Check sheet for the modelled part. Datum: model origin and axes. Units: mm. Face numbers are marked on the shaded views. A direction names the side the tool comes from. Give positions to 0.01 mm unless a question says otherwise; leave off trailing zeros. Loops run counter-clockwise (first coordinate to the right, second up) from the corner with the lowest first, then second, coordinate; pieces in that order, holes last.
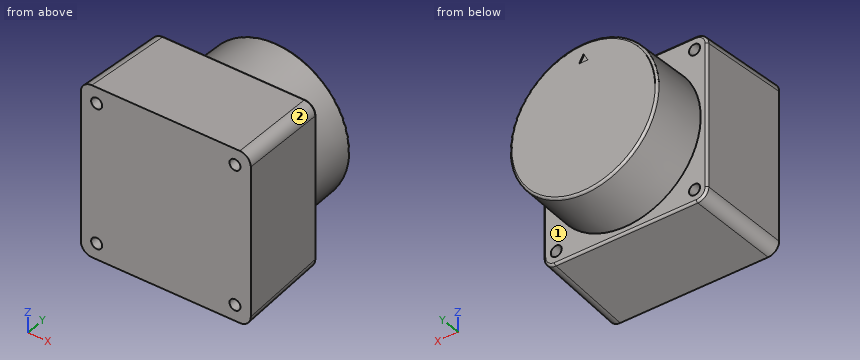
```python
from build123d import *

# Parameters (mm, degrees)
SZKIC1_W                    = 38.59
SZKIC1_H                    = 38.59
SZKIC1_R                    = 1.25
DODANIE_WYCI_GNI_CIE1_DEPTH = 33.3
SZKIC3_OUTSIDE_W            = 53.376
SZKIC3_OUTSIDE_H            = 53.376
SZKIC3_OUTSIDE_R            = 17.645
WYTNIJ_WYCI_GNI_CIE1_DEPTH  = 12.6
POCHYLENIE2_ANGLE           = -2
POCHYLENIE3_ANGLE           = -1.5
ZAOKR_GLENIE2_R             = 2.5
ZAOKR_GLENIE3_R             = 0.5
ZAOKR_GLENIE4_R             = 0.5
WYTNIJ_WYCI_GNI_CIE2_DEPTH  = 0.2


with BuildPart() as part:
    # Szkic1 → Dodanie-wyciągnięcie1 (new body)
    with BuildSketch(Plane(origin=(0, 0, 0), x_dir=(1, 0, 0), z_dir=(0, 1, 0))):
        Rectangle(SZKIC1_W, SZKIC1_H)
        with Locations(Location((-15.7, 15.7, 0), (0, 0, 270))):
            Circle(SZKIC1_R, mode=Mode.SUBTRACT)
        with Locations(Location((15.7, 15.7, 0), (0, 0, 270))):
            Circle(SZKIC1_R, mode=Mode.SUBTRACT)
        with Locations(Location((15.7, -15.7, 0), (0, 0, 270))):
            Circle(SZKIC1_R, mode=Mode.SUBTRACT)
        with Locations(Location((-15.7, -15.7, 0), (0, 0, 270))):
            Circle(SZKIC1_R, mode=Mode.SUBTRACT)
    extrude(amount=DODANIE_WYCI_GNI_CIE1_DEPTH)

    # Szkic3 outside → Wytnij-wyciągnięcie1 (cut)
    with BuildSketch(Plane(origin=(0, 33.3, 0), x_dir=(1, 0, 0), z_dir=(0, 1, 0))):
        Rectangle(SZKIC3_OUTSIDE_W, SZKIC3_OUTSIDE_H)
        with Locations(Location((0, 0, 0), (0, 0, 270))):
            Circle(SZKIC3_OUTSIDE_R, mode=Mode.SUBTRACT)
    extrude(amount=-WYTNIJ_WYCI_GNI_CIE1_DEPTH, mode=Mode.SUBTRACT)

    # Pochylenie2
    pochylenie2_faces = [part.faces().sort_by_distance(p)[0] for p in [
        (19.295, 10.35, 0),
        (0, 10.35, 19.295),
        (-19.295, 10.35, 0),
        (0, 10.35, -19.295),
    ]]
    draft(pochylenie2_faces, Plane(origin=(0, 0, 0), x_dir=(0, 0, -1), z_dir=(0, -1, 0)), POCHYLENIE2_ANGLE)

    # Pochylenie3
    pochylenie3_faces = [part.faces().sort_by_distance(p)[0] for p in [
        (0, 27, -17.645),
    ]]
    draft(pochylenie3_faces, Plane(origin=(0, 0, 0), x_dir=(0, 0, -1), z_dir=(0, -1, 0)), POCHYLENIE3_ANGLE)

    # Zaokrąglenie2
    zaokr_glenie2_edges = [part.edges().sort_by_distance(p)[0] for p in [
        (18.933570036, 10.35, 18.933570036),
        (-18.933570036, 10.35, 18.933570036),
        (-18.933570036, 10.35, -18.933570036),
        (18.933570036, 10.35, -18.933570036),
    ]]
    fillet(zaokr_glenie2_edges, radius=ZAOKR_GLENIE2_R)

    # Zaokrąglenie3
    zaokr_glenie3_edges = [part.edges().sort_by_distance(p)[0] for p in [
        (0, 20.7, -18.572140072),
        (18.572140072, 20.7, 0),
        (-18.572140072, 20.7, 0),
        (0, 20.7, 18.572140072),
        (17.840537572, 20.7, 17.840537572),
        (-17.840537572, 20.7, 17.840537572),
        (-17.840537572, 20.7, -17.840537572),
        (17.840537572, 20.7, -17.840537572),
    ]]
    fillet(zaokr_glenie3_edges, radius=ZAOKR_GLENIE3_R)

    # Zaokrąglenie4
    zaokr_glenie4_edges = [part.edges().sort_by_distance(p)[0] for p in [
        (0, 33.3, -16.773008812),
    ]]
    fillet(zaokr_glenie4_edges, radius=ZAOKR_GLENIE4_R)

    # Szkic4 → Wytnij-wyciągnięcie2 (cut)
    with BuildSketch(Plane(origin=(0, 33.3, 0), x_dir=(1, 0, 0), z_dir=(0, 1, 0))):
        Polygon((-1, -12.549966068), (1, -12.549966068), (0, -14.282016876), align=None)
    extrude(amount=-WYTNIJ_WYCI_GNI_CIE2_DEPTH, mode=Mode.SUBTRACT)


solid = part.part
```
(1) Section check B-B on y = 19.5. Give the number of separate pieces and of enclosed holes in the cut face, plus the area to 3 significant figures.
(2) Gauge pin test, flat ends, axial feed: pin 1 Ø6 at (y, z) = (11.5, 15.5) entering from +X; pin 2 Ø1 at (y, z) = (26.5, 9) entering from -X; pin 3 Ø6 at (x, y) = (10, 22) entering from +Z; pin 4 Ø1.5 at (x, z) = (15.7, -15.7) entering from +Y (3 decimals). Record the tip position at first contact, or that the pin passes through.
(3) Material ranges on line 1 (X direction, y = 4, z = -15); line 2 (Z direction, x = 15, y = 15); line 3 (X direction, y = 9, z = 15), recorded low to high.
(4) Section check C-C on y = 29. Record the boundary of the cut face in (x, z).
(5) Access from +Z, -Z, +X, -X, +Y, -Y to the whole of each face (thin tool, end or side, straight path). Record for the marked faces 1 and 2.
(6) Section check A-A on z = 0. Record the boundary of the cut face in (x, y) (3 decimals).
(7) Section check D-D on y = 24. Record the boundary of the cut face in (x, z), plus the area to 3 significant figures.
Computed values:
1. separate pieces: 1
1. enclosed holes: 4
1. area: 1,360 mm2
2. pin 1: stops at x = 19
2. pin 2: stops at x = -14.67
2. pin 3: stops at z = 18.63
2. pin 4: passes through
3. line 1: x = -19.16 to -16.74, -14.66 to 14.66, 16.74 to 19.16
3. line 2: z = -18.77 to -16.74, -14.66 to 14.66, 16.74 to 18.77
3. line 3: x = -18.98 to -16.74, -14.66 to 14.66, 16.74 to 18.98
4. outline: circle Ø33.77 at (0, 0)
5. face 1: +Y
5. face 2: +Z, +X, +Y
6. outline: (-19.295, 0) - (19.295, 0) - (18.589, 20.217) arc R0.5 ccw to (18.089, 20.7) - (17.103, 20.7) - (16.786, 32.813) arc R0.5 ccw to (16.286, 33.3) - (-16.286, 33.3) arc R0.5 ccw to (-16.786, 32.813) - (-17.103, 20.7) - (-18.089, 20.7) arc R0.5 ccw to (-18.589, 20.217) - close
7. outline: circle Ø34.03 at (0, 0)
7. area: 910 mm2
